Geometry: final body of the model. Coordinates: model frame, mm. A direction names the side the tool comes from. Give positions to 0.01 mm unless a question says otherwise; leave off trailing zeros. Write each loop counter-clockwise with the first axis right and the second up, starting at its lowest first coordinate (ties: lowest second). Pieces come first, ordered by that corner, then holes. Notation, with made-up numbers: (84.25, 25) -> (109.25, 25) arc R28 cw to (109.25, 43) -> close; hole circle Ø3 at (69, 58). An arc over 180 degrees is marked (long way). Answer in a Markdown table with one row per item. Add a question column.
Item 1: Draft query along Z for faces 5 (the flat face through (-1, 31, 0)), 6 (the flat face through (-1, 33, -5.6)), 7 (the flat face through (-1, 31, -40.2)). Return one class per face: +Z half, -Z half, draft (parallel to the pull), parting line (faces both ways), or undercut.
Item 2: Material intervals for probe 1 along Y at (x, z) = (-0.55, -37.4); probe 2 along Z at (x, y) = (-0.7, 45); probe 3 along X at (y, z) = (15, -4), sorted ascending. Write a range as from..to.
Item 3: Access query for faces 1 (the cylindrical face through (-0.74, 50.78, -2.51)), 2 (the flat face through (-1, 4.3, -20)), 3 (the flat face through (-1, 33, -34.6)), 4 (the flat face through (0, 34, -37)). Directions: +Z, -Z, +X, -X, +Y, -Y. A direction counts if a zero-diameter tool reaches every point of the face in a straight line with its end or side. Return the directions, or none.
Item 4: Section query A-A on z = -31.1. Output: boundary loops of the cut face in (x, y), plus the area to 3 significant figures.
Item 5: First-contact query: P1, Ø3, axis at y = 2.8, z = -9.1, coming from the +X side; P2, Ø3.5, axis at y = 52.1, z = -37.4, coming from the +X side; P3, Ø0.6, axis at x = -0.5, z = -14, coming from the +Y side; P4, Ø2, axis at y = 2.5, z = -22.5, coming from the -X side. Flat tips, straight axial feed; report the tip coordinate or a pass-through.
Item 6: Section query B-B on y = 13. Output: boundary loops of the cut face in (x, z), plus the area to 3 significant figures.
Item 7: Section query C-C on z = -2.8. Output: boundary loops of the cut face in (x, y), plus the area to 3 significant figures.
Item 8: Section query D-D on z = -22. Output: boundary loops of the cut face in (x, y), plus the area to 3 significant figures.
```python
from build123d import *

# Parameters (mm, degrees)
BOSS_EXTRUDE1_DEPTH = 40.2
CUT_EXTRUDE2_REACH  = 3.5
SKETCH3_R           = 1.35
SKETCH3_W           = 29
SKETCH3_H           = 55.3
FILLET1_R           = 1
CUT_EXTRUDE3_REACH  = 5
SKETCH4_R           = 1.35


with BuildPart() as part:
    # Sketch1 → Boss-Extrude1 (new body)
    with BuildSketch(Plane.XY):
        Polygon((0, 0), (0, 4.3), (-1.5, 4.3), (-1.5, 61.1), (0, 61.1), (0, 5.8), (1.5, 5.8), (1.5, 0), align=None)
    extrude(amount=-BOSS_EXTRUDE1_DEPTH)

    # Sketch3 → Cut-Extrude2 (cut, up to next)
    with BuildSketch(Plane(origin=(0, 0, 0), x_dir=(0, 0, -1), z_dir=(1, 0, 0)), mode=Mode.PRIVATE) as cut_extrude2_sk1:
        with Locations((2.8, 8.1)):
            Circle(SKETCH3_R)
    cut_extrude2_tool1 = extrude(cut_extrude2_sk1.sketch, amount=-CUT_EXTRUDE2_REACH, mode=Mode.PRIVATE) & part.part
    add(cut_extrude2_tool1.solids().sort_by_distance((0, 8.1, -2.8))[0], mode=Mode.SUBTRACT)
    # Sketch3 → Cut-Extrude2 (cut, up to next)
    with BuildSketch(Plane(origin=(0, 0, 0), x_dir=(0, 0, -1), z_dir=(1, 0, 0)), mode=Mode.PRIVATE) as cut_extrude2_sk2:
        with Locations((37.4, 8.1)):
            Circle(SKETCH3_R)
    cut_extrude2_tool2 = extrude(cut_extrude2_sk2.sketch, amount=-CUT_EXTRUDE2_REACH, mode=Mode.PRIVATE) & part.part
    add(cut_extrude2_tool2.solids().sort_by_distance((0, 8.1, -37.4))[0], mode=Mode.SUBTRACT)
    # Sketch3 → Cut-Extrude2 (cut, up to next)
    with BuildSketch(Plane(origin=(0, 0, 0), x_dir=(0, 0, -1), z_dir=(1, 0, 0)), mode=Mode.PRIVATE) as cut_extrude2_sk3:
        with Locations((2.8, 30.1)):
            Circle(SKETCH3_R)
    cut_extrude2_tool3 = extrude(cut_extrude2_sk3.sketch, amount=-CUT_EXTRUDE2_REACH, mode=Mode.PRIVATE) & part.part
    add(cut_extrude2_tool3.solids().sort_by_distance((0, 30.1, -2.8))[0], mode=Mode.SUBTRACT)
    # Sketch3 → Cut-Extrude2 (cut, up to next)
    with BuildSketch(Plane(origin=(0, 0, 0), x_dir=(0, 0, -1), z_dir=(1, 0, 0)), mode=Mode.PRIVATE) as cut_extrude2_sk4:
        with Locations((37.4, 30.1)):
            Circle(SKETCH3_R)
    cut_extrude2_tool4 = extrude(cut_extrude2_sk4.sketch, amount=-CUT_EXTRUDE2_REACH, mode=Mode.PRIVATE) & part.part
    add(cut_extrude2_tool4.solids().sort_by_distance((0, 30.1, -37.4))[0], mode=Mode.SUBTRACT)
    # Sketch3 → Cut-Extrude2 (cut, up to next)
    with BuildSketch(Plane(origin=(0, 0, 0), x_dir=(0, 0, -1), z_dir=(1, 0, 0)), mode=Mode.PRIVATE) as cut_extrude2_sk5:
        with Locations((2.8, 52.1)):
            Circle(SKETCH3_R)
    cut_extrude2_tool5 = extrude(cut_extrude2_sk5.sketch, amount=-CUT_EXTRUDE2_REACH, mode=Mode.PRIVATE) & part.part
    add(cut_extrude2_tool5.solids().sort_by_distance((0, 52.1, -2.8))[0], mode=Mode.SUBTRACT)
    # Sketch3 → Cut-Extrude2 (cut, up to next)
    with BuildSketch(Plane(origin=(0, 0, 0), x_dir=(0, 0, -1), z_dir=(1, 0, 0)), mode=Mode.PRIVATE) as cut_extrude2_sk6:
        with Locations((37.4, 52.1)):
            Circle(SKETCH3_R)
    cut_extrude2_tool6 = extrude(cut_extrude2_sk6.sketch, amount=-CUT_EXTRUDE2_REACH, mode=Mode.PRIVATE) & part.part
    add(cut_extrude2_tool6.solids().sort_by_distance((0, 52.1, -37.4))[0], mode=Mode.SUBTRACT)
    # Sketch3 → Cut-Extrude2 (cut, up to next)
    with BuildSketch(Plane(origin=(0, 0, 0), x_dir=(0, 0, -1), z_dir=(1, 0, 0)), mode=Mode.PRIVATE) as cut_extrude2_sk7:
        with Locations((20.1, 33.45)):
            Rectangle(SKETCH3_W, SKETCH3_H)
    cut_extrude2_tool7 = extrude(cut_extrude2_sk7.sketch, amount=-CUT_EXTRUDE2_REACH, mode=Mode.PRIVATE) & part.part
    add(cut_extrude2_tool7.solids().sort_by_distance((0, 33.45, -20.1))[0], mode=Mode.SUBTRACT)

    # Fillet1
    fillet1_edges = [part.edges().sort_by_distance(p)[0] for p in [
        (1.5, 5.8, -20.1),
    ]]
    fillet(fillet1_edges, radius=FILLET1_R)

    # Sketch4 → Cut-Extrude3 (cut, up to next)
    with BuildSketch(Plane(origin=(1.5, 0, 0), x_dir=(0, 0, -1), z_dir=(1, 0, 0)), mode=Mode.PRIVATE) as cut_extrude3_sk1:
        with Locations((9.1, 2.8)):
            Circle(SKETCH4_R)
    cut_extrude3_tool1 = extrude(cut_extrude3_sk1.sketch, amount=-CUT_EXTRUDE3_REACH, mode=Mode.PRIVATE) & part.part
    add(cut_extrude3_tool1.solids().sort_by_distance((1.5, 2.8, -9.1))[0], mode=Mode.SUBTRACT)
    # Sketch4 → Cut-Extrude3 (cut, up to next)
    with BuildSketch(Plane(origin=(1.5, 0, 0), x_dir=(0, 0, -1), z_dir=(1, 0, 0)), mode=Mode.PRIVATE) as cut_extrude3_sk2:
        with Locations((31.1, 2.8)):
            Circle(SKETCH4_R)
    cut_extrude3_tool2 = extrude(cut_extrude3_sk2.sketch, amount=-CUT_EXTRUDE3_REACH, mode=Mode.PRIVATE) & part.part
    add(cut_extrude3_tool2.solids().sort_by_distance((1.5, 2.8, -31.1))[0], mode=Mode.SUBTRACT)


solid = part.part
```
Findings below:
| question | item | result |
|---|---|---|
| 1 | face 5 | +Z half |
| 1 | face 6 | undercut |
| 1 | face 7 | -Z half |
| 2 | probe 1 | y = 4.3..6.75, 9.45..28.75, 31.45..50.75, 53.45..61.1 |
| 2 | probe 2 | z = -40.2..-34.6, -5.6..0 |
| 2 | probe 3 | x = -1.5..0 |
| 3 | face 1 | +X, -X |
| 3 | face 2 | +Z, -Z, -X, -Y |
| 3 | face 3 | +X, -X, +Y |
| 3 | face 4 | +Z, -Z, +X, +Y |
| 4 | outline | (-1.5, 4.3) -> (0, 4.3) -> (0, 4.15) -> (1.5, 4.15) -> (1.5, 4.8) arc R1 ccw to (0.5, 5.8) -> (-1.5, 5.8) -> close; (0, 0) -> (1.5, 0) -> (1.5, 1.45) -> (0, 1.45) -> close |
| 4 | area | 6.69 mm^2 |
| 5 | P1 | stops at x = 1.5 |
| 5 | P2 | stops at x = 0 |
| 5 | P3 | stops at y = 5.8 |
| 5 | P4 | stops at x = 0 |
| 6 | outline | (-1.5, -40.2) -> (0, -40.2) -> (0, -34.6) -> (-1.5, -34.6) -> close; (-1.5, -5.6) -> (0, -5.6) -> (0, 0) -> (-1.5, 0) -> close |
| 6 | area | 16.8 mm^2 |
| 7 | outline | (-1.5, 4.3) -> (0, 4.3) -> (0, 0) -> (1.5, 0) -> (1.5, 4.8) arc R1 ccw to (0.5, 5.8) -> (0, 5.8) -> (0, 6.75) -> (-1.5, 6.75) -> close; (-1.5, 9.45) -> (0, 9.45) -> (0, 28.75) -> (-1.5, 28.75) -> close; (-1.5, 31.45) -> (0, 31.45) -> (0, 50.75) -> (-1.5, 50.75) -> close; (-1.5, 53.45) -> (0, 53.45) -> (0, 61.1) -> (-1.5, 61.1) -> close |
| 7 | area | 81.5 mm^2 |
| 8 | outline | (-1.5, 4.3) -> (0, 4.3) -> (0, 0) -> (1.5, 0) -> (1.5, 4.8) arc R1 ccw to (0.5, 5.8) -> (-1.5, 5.8) -> close |
| 8 | area | 10.7 mm^2 |
